Check sheet for the modelled part. Datum: model origin and axes. Units: mm. Face numbers are marked on the shaded views. Give positions to 0.01 mm unless a question says otherwise; leave off trailing zeros. Write each loop counter-clockwise with the first axis right and the second up, starting at its lowest first coordinate (ties: lowest second). Pieces come first, ordered by that corner, then holes. Notation, with made-up numbers: M -28.5,-10.75 L -1.5,-10.75 A13 ccw -1.5,7.25 Z; hole C 37.5,-10 d10. An arc over 180 degrees is marked long. Use CSV: the item, a comma, the result in double quotes. Start each with the question number.
1. Cross-section at C-C, the plane y = -13.75. Enter the section's corners in (x, z) (3 decimals).
2. Mould release check, pull along Z, two halves, no side actions. Record for the marked faces 1 and 2: +Z half, -Z half, draft (parallel to the pull), parting line (faces both ways), or undercut.
3. Depth check by flat-ended pin: P1, Ø4, axis at y = -8.5, z = -123, coming from the +X side (3 decimals); P2, Ø10.5, axis at y = -10.5, z = -317.5, coming from the +X side; P3, Ø5, axis at x = 84.5, y = -4, coming from the +Z side; P4, Ø10, axis at x = 41.5, z = -83.5, coming from the -Y side. Enter the tip coordinate at first touch or a pass-through.
4. Scan lines: line 1 (Z direction, x = 114, y = -1.5) (1 decimal); line 2 (X direction, y = -5, z = -336) (3 decimals); line 3 (X direction, y = -17, z = -122.5) (3 decimals). Record each from-to range of solid material in increasing order.
from build123d import *

# Parameters (mm, degrees)
SKETCH1_W           = 152.4
SKETCH1_H           = 457.2
BOSS_EXTRUDE1_DEPTH = 3.175
SKETCH2_W           = 3.175
SKETCH2_H           = 457.2
BOSS_EXTRUDE2_DEPTH = 23.8125
SKETCH3_W           = 133.35
SKETCH3_H           = 3.175
BOSS_EXTRUDE3_DEPTH = 6.35
SKETCH9_W           = 3.175
SKETCH9_H           = 457.2
BOSS_EXTRUDE4_DEPTH = 6.35
SKETCH11_R          = 6.35
CUT_EXTRUDE1_DEPTH  = 483.519051599


with BuildPart() as part:
    # Sketch1 → Boss-Extrude1 (new body)
    with BuildSketch(Plane(origin=(0, 0, 0), x_dir=(1, 0, 0), z_dir=(0, 1, 0))):
        with Locations((76.2, 228.6)):
            Rectangle(SKETCH1_W, SKETCH1_H)
    extrude(amount=BOSS_EXTRUDE1_DEPTH)

    # Sketch2 → Boss-Extrude2 (add)
    with BuildSketch(Plane(origin=(0, 3.175, 0), x_dir=(1, 0, 0), z_dir=(0, 1, 0))):
        with Locations((1.5875, 228.6)):
            Rectangle(SKETCH2_W, SKETCH2_H)
    extrude(amount=-BOSS_EXTRUDE2_DEPTH)

    # Sketch3 → Boss-Extrude3 (add)
    with BuildSketch(Plane.XZ):
        with Locations((66.675, -107.95)):
            Rectangle(SKETCH3_W, SKETCH3_H)
        with Locations((66.675, -228.6)):
            Rectangle(SKETCH3_W, SKETCH3_H)
        with Locations((66.675, -349.25)):
            Rectangle(SKETCH3_W, SKETCH3_H)
        with Locations((66.675, -1.5875)):
            Rectangle(SKETCH3_W, SKETCH3_H)
        with Locations((66.675, -455.6125)):
            Rectangle(SKETCH3_W, SKETCH3_H)
    extrude(amount=BOSS_EXTRUDE3_DEPTH)

    # Sketch9 → Boss-Extrude4 (add)
    with BuildSketch(Plane.XZ):
        with Locations((131.7625, -228.6)):
            Rectangle(SKETCH9_W, SKETCH9_H)
    extrude(amount=BOSS_EXTRUDE4_DEPTH)

    # Sketch11 → Cut-Extrude1 (cut, through all)
    with BuildSketch(Plane(origin=(0, 3.175, 0), x_dir=(1, 0, 0), z_dir=(0, 1, 0))):
        with Locations((152.4, 228.6)):
            Circle(SKETCH11_R)
    extrude(amount=-CUT_EXTRUDE1_DEPTH, mode=Mode.SUBTRACT)


solid = part.part
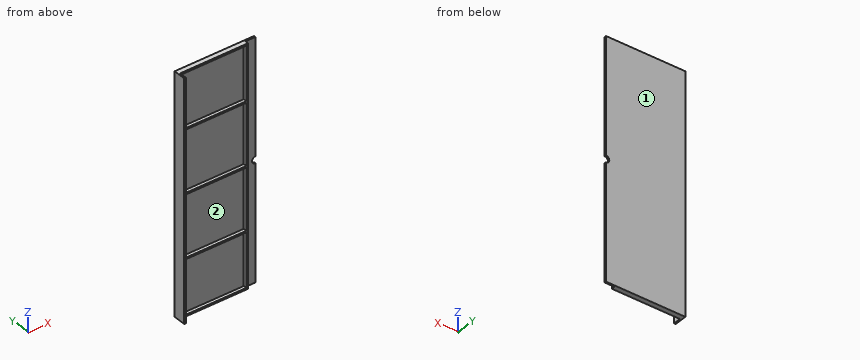
Worked answers:
1,outline,"M 0,-457.2 L 3.175,-457.2 L 3.175,0 L 0,0 Z"
2,face 1,"draft"
2,face 2,"undercut"
3,P1,"stops at x = 3.175"
3,P2,"stops at x = 133.35"
3,P3,"stops at z = 0"
3,P4,"stops at y = 0"
4,line 1,"z = -457.2 to -454, -350.8 to -347.7, -230.2 to -227, -109.5 to -106.4, -3.2 to 0"
4,line 2,"x = 0 to 3.175, 130.175 to 133.35"
4,line 3,"x = 0 to 3.175"
